from build123d import *

# Parameters (mm, degrees)
F0_R     = 9
F1_DEPTH = 25
F2_W     = 8
F2_H     = 8
F3_DEPTH = 10
F4_W     = 8
F4_H     = 36
F5_DEPTH = 6
F6_R     = 3


with BuildPart() as f1:
    # F0 (on Top) → F1 (new body)
    with BuildSketch(Plane.XY):
        Circle(F0_R)
    extrude(amount=F1_DEPTH)

    # F2 (on face) → F3 (cut)
    with BuildSketch(Plane(origin=(0, 0, 0), x_dir=(1, 0, 0), z_dir=(0, 0, -1))):
        Rectangle(F2_W, F2_H)
    extrude(amount=-F3_DEPTH, mode=Mode.SUBTRACT)

    # F4 (on face) → F5 (join, symmetric)
    with BuildSketch(Plane.XY.offset(25)):
        Rectangle(F4_W, F4_H)
    extrude(amount=F5_DEPTH, both=True)

    # F6
    f6_edges = [f1.edges().sort_by_distance(p)[0] for p in [
        (-4, 18, 25),
        (4, 18, 25),
        (-4, -18, 25),
        (4, -18, 25),
        (-4, 0, 25),
        (-4, -8.062258, 22),
        (-4, 8.062258, 22),
        (4, -8.062258, 22),
        (4, 8.062258, 22),
        (4, 0, 25),
    ]]
    fillet(f6_edges, radius=F6_R)


solid = f1.part
Verification items for the finished model (mm, model axes). A direction names the side the tool comes from. Round coordinates to 2 decimals unless told otherwise and drop trailing zeros. Loops run counter-clockwise (first coordinate to the right, second up) from the corner with the lowest first, then second, coordinate; pieces in that order, holes last. Notation, with made-up numbers: (-5, 26.25) - (25, 26.25) arc R27 cw to (25, 43.25) - close; hole circle Ø4 at (13, 41). An arc over 180 degrees is marked (long way). Write item = value, one per line.
Q1. Sectioned sample at C-C on x = 0. Record the boundary of the cut face in (y, z).
Here are the results:
outline = (-18, 19) - (-9, 19) - (-9, 0) - (-4, 0) - (-4, 10) - (4, 10) - (4, 0) - (9, 0) - (9, 19) - (18, 19) - (18, 31) - (-18, 31) - close
Q2. Tool access check on faces 1 (the flat face through (4, 0, 29)), 2 (the flat face through (0, -4, 5)), 3 (the flat face through (-8, 0, 25)), 4 (the flat face through (-4, 0, 29)). Record the directions out of +Z, -Z, +X, -X, +Y, -Y that give a thin tool (end or side, any length) a straight path to the whole face; none if there is none.
Here are the results:
face_1 = +Z, +X
face_2 = -Z
face_3 = +Z, -X, +Y, -Y
face_4 = +Z, -X
Q3. Depth check by flat-ended pin: pin 1 (1 mm diameter, centred on x = 0.5, z = 11.5, fed in from +Y); pin 2 (2 mm diameter, centred on x = 6, y = 10, fed in from -Z); pin 3 (3 mm diameter, centred on x = -7, z = 11, fed in from +Y); pin 4 (9 mm diameter, centred on x = 0.5, z = 5, fed in from -Y). Enter the tip coordinate at first touch or a pass-through.
Here are the results:
pin_1 = 9
pin_2 = through
pin_3 = 7.12
pin_4 = -9
Q4. Mould release check, pull along Y, two halves, no side actions. Record for faces 5 (the flat face through (0, -13, 19)), 6 (the flat face through (0, -18, 25)), 7 (the flat face through (4, 0, 5)): +Y half, -Y half, draft (parallel to the pull), parting line (faces both ways), or undercut.
Here are the results:
face_5 = draft
face_6 = -Y half
face_7 = undercut
Q5. Material ranges on L1, parallel to Y at x = 5.25, z = 22; L2, parallel to Y at x = -3.5, z = 6; L3, parallel to X at y = -0.5, z = 14.5, recorded low to high.
Here are the results:
L1 = -7.31 to 7.31
L2 = -8.29 to -4, 4 to 8.29
L3 = -8.99 to 8.99
Q6. Sectioned sample at B-B on y = 0. Record the boundary of the cut face in (x, z).
Here are the results:
outline = (-9, 0) - (-4, 0) - (-4, 10) - (4, 10) - (4, 0) - (9, 0) - (9, 25) - (7, 25) arc R3 cw to (4, 28) - (4, 31) - (-4, 31) - (-4, 28) arc R3 cw to (-7, 25) - (-9, 25) - close
Q7. Sectioned sample at D-D on x = -2. Record the boundary of the cut face in (y, z), plus the area to 3 significant figures.
Here are the results:
outline = (-17.83, 19) - (-8.77, 19) - (-8.77, 0) - (-4, 0) - (-4, 10) - (4, 10) - (4, 0) - (8.77, 0) - (8.77, 19) - (17.83, 19) - (17.83, 31) - (-17.83, 31) - close
area = 681 mm^2
Q8. Sectioned sample at A-A on z = 20. Record the boundary of the cut face in (x, y), plus the area to 3 significant figures.
Here are the results:
outline = (-5.25, -7.31) arc R3 cw to (-4, -9.75) - (-4, -15) arc R3 ccw to (-1, -18) - (1, -18) arc R3 ccw to (4, -15) - (4, -9.75) arc R3 cw to (5.25, -7.31) arc R9 ccw to (5.25, 7.31) arc R3 cw to (4, 9.75) - (4, 15) arc R3 ccw to (1, 18) - (-1, 18) arc R3 ccw to (-4, 15) - (-4, 9.75) arc R3 cw to (-5.25, 7.31) arc R9 ccw to start
area = 397 mm^2
